from build123d import *

# Parameters (mm, degrees)
SKETCH1_R                      = 7.5
BOSS_EXTRUDE1_DEPTH            = 17
CUT_EXTRUDE1_REACH             = 45.661
SKETCH2_R                      = 2.5
CUT_EXTRUDE1_DIRECTION_2_DEPTH = 44.660622991
FILLET1_R                      = 5
FILLET2_R                      = 5


with BuildPart() as part:
    # Sketch1 → Boss-Extrude1 (new body)
    with BuildSketch(Plane.XY):
        with BuildLine():
            Line((-25, 19), (25, 19))
            Line((25, 19), (25, 7.5))
            Line((25, 7.5), (10, 7.5))
            ThreePointArc((10, 7.5), (0, -12.5), (-10, 7.5))
            Line((-10, 7.5), (-25, 7.5))
            Line((-25, 7.5), (-25, 19))
        make_face()
        Circle(SKETCH1_R, mode=Mode.SUBTRACT)
    extrude(amount=BOSS_EXTRUDE1_DEPTH)

    # Sketch2 → Cut-Extrude1 (cut, up to next)
    with BuildSketch(Plane(origin=(0, 19, 0), x_dir=(1, 0, 0), z_dir=(0, 1, 0)), mode=Mode.PRIVATE) as cut_extrude1_sk1:
        with Locations(Location((20, -8.5, 0), (0, 0, 90))):
            Circle(SKETCH2_R)
    cut_extrude1_tool1 = extrude(cut_extrude1_sk1.sketch, amount=-CUT_EXTRUDE1_REACH, mode=Mode.PRIVATE) & part.part
    # Sketch2 → Cut-Extrude1 (cut, up to next)
    with BuildSketch(Plane(origin=(0, 19, 0), x_dir=(1, 0, 0), z_dir=(0, 1, 0)), mode=Mode.PRIVATE) as cut_extrude1_sk2:
        with Locations(Location((-20, -8.5, 0), (0, 0, 90))):
            Circle(SKETCH2_R)
    cut_extrude1_tool2 = extrude(cut_extrude1_sk2.sketch, amount=-CUT_EXTRUDE1_REACH, mode=Mode.PRIVATE) & part.part
    add(cut_extrude1_tool1.solids().sort_by_distance((20, 19, 8.5))[0], mode=Mode.SUBTRACT)
    add(cut_extrude1_tool2.solids().sort_by_distance((-20, 19, 8.5))[0], mode=Mode.SUBTRACT)

    # Sketch2 → Cut-Extrude1 direction 2 (cut)
    with BuildSketch(Plane(origin=(0, 19, 0), x_dir=(1, 0, 0), z_dir=(0, 1, 0))):
        with Locations(Location((20, -8.5, 0), (0, 0, 90))):
            Circle(SKETCH2_R)
        with Locations(Location((-20, -8.5, 0), (0, 0, 90))):
            Circle(SKETCH2_R)
    extrude(amount=CUT_EXTRUDE1_DIRECTION_2_DEPTH, mode=Mode.SUBTRACT)

    # Fillet1
    fillet1_edges = [part.edges().sort_by_distance(p)[0] for p in [
        (-10, 7.5, 8.5),
    ]]
    fillet(fillet1_edges, radius=FILLET1_R)

    # Fillet2
    fillet2_edges = [part.edges().sort_by_distance(p)[0] for p in [
        (10, 7.5, 8.5),
    ]]
    fillet(fillet2_edges, radius=FILLET2_R)


solid = part.part
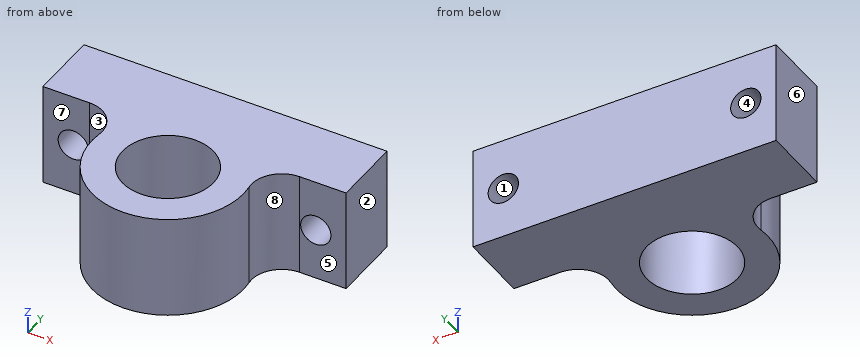
Verification items for the finished model (mm, model axes). Face numbers are marked on the shaded views. A direction names the side the tool comes from. Coordinates: 2 decimals unless noted, no trailing zeros. Write each loop counter-clockwise with the first axis right and the second up, starting at its lowest first coordinate (ties: lowest second). Pieces come first, ordered by that corner, then holes. Notation, with made-up numbers: M -40,36.5 L 15,36.5 A28 ccw 15,74.5 Z; hole C -17.5,-1 d3. An arc over 180 degrees is marked long. Use a Markdown table: item, result.
Q1. Go/stop test with flat-tipped pins: P1, Ø1, axis at y = -3.5, z = 11.5, coming from the -X side; P2, Ø3, axis at x = 20, z = 8.5, coming from the +Y side; P3, Ø2, axis at x = -3.5, z = 4.5, coming from the -Y side; P4, Ø3, axis at y = -2, z = 8, coming from the +X side. Record where each tip stops, or that it passes through.
Reply:
| item | result |
|---|---|
| P1 | stops at x = -12.13 |
| P2 | passes through |
| P3 | stops at y = -12.25 |
| P4 | stops at x = 12.49 |
Q2. Set-up check for the marked faces 5, 6, 7 and 8: record each of +Z, -Z, +X, -X, +Y, -Y from which the full face is reachable in a straight line by a thin tool's end or side.
Reply:
| item | result |
|---|---|
| face 5 | +Z, -Z, +X, -Y |
| face 6 | +Z, -Z, -X, +Y, -Y |
| face 7 | +Z, -Z, -X, -Y |
| face 8 | +Z, -Z, +X |
Q3. Sectioned sample at B-B, the plane x = 0. Record the boundary of the cut face in (y, z), plus the area to 4 significant figures.
Reply:
| item | result |
|---|---|
| outline | M -12.5,0 L -7.5,0 L -7.5,17 L -12.5,17 Z; M 7.5,0 L 19,0 L 19,17 L 7.5,17 Z |
| area | 280.5 mm² |
Q4. Draft check along X on the marked faces 1, 2, 3 and 4. Enter one of: +X half, -X half, draft (parallel to the pull), parting line (faces both ways), or undercut.
Reply:
| item | result |
|---|---|
| face 1 | undercut |
| face 2 | +X half |
| face 3 | -X half |
| face 4 | undercut |
Q5. Sectioned sample at A-A, the plane z = 8.25. Record the boundary of the cut face in (x, y).
Reply:
| item | result |
|---|---|
| outline | M -25,7.5 L -22.49,7.5 L -22.49,19 L -25,19 Z; M -17.51,7.5 L -17.32,7.5 A5 cw -12.37,1.79 A12.5 ccw long 12.37,1.79 A5 cw 17.32,7.5 L 17.51,7.5 L 17.51,19 L -17.51,19 Z; M 22.49,7.5 L 25,7.5 L 25,19 L 22.49,19 Z; hole C 0,0 d15 |
Q6. Sectioned sample at D-D, the plane z = 12.75. Record the boundary of the cut face in (x, y), plus the area to 3 significant figures.
Reply:
| item | result |
|---|---|
| outline | M -25,7.5 L -17.32,7.5 A5 cw -12.37,1.79 A12.5 ccw long 12.37,1.79 A5 cw 17.32,7.5 L 25,7.5 L 25,19 L -25,19 Z; hole C 0,0 d15 |
| area | 840 mm² |
Q7. Thickness scan on line 1 (X direction, y = 10, z = 8.5); line 2 (Z direction, x = -20, y = 10); line 3 (X direction, y = 3, z = 8). Record the ranges inside material, lowest first.
Reply:
| item | result |
|---|---|
| line 1 | x = -25 to -22.5, -17.5 to 17.5, 22.5 to 25 |
| line 2 | z = 0 to 6, 11 to 17 |
| line 3 | x = -12.35 to -6.87, 6.87 to 12.35 |
Q8. Sectioned sample at C-C, the plane y = 0. Record the boundary of the cut face in (x, z), plus the area to 3 significant figures.
Reply:
| item | result |
|---|---|
| outline | M -12.5,0 L -7.5,0 L -7.5,17 L -12.5,17 Z; M 7.5,0 L 12.5,0 L 12.5,17 L 7.5,17 Z |
| area | 170 mm² |
